Here's how the part is built. I have some questions about the finished solid (model axes, mm). Round coordinates to 2 decimals unless told otherwise and drop trailing zeros. Use a Markdown table: item, result. Add a question column.
(1) I'm going to push flat-ended pins straight in: P1, Ø5, axis at x = -11.5, y = 3.5, coming from the -Z side; P2, Ø0.9, axis at x = -13, z = -358.5, coming from the +Y side; P3, Ø1.9, axis at y = -30, z = -457.5, coming from the +X side. Where does each tip first touch, or does it pass through?
(2) If I drill on probe 1 along Y at (x, z) = (0, 13); probe 2 along Y at (x, z) = (0.75, -193); probe 3 along Y at (x, z) = (7.25, -418.5), over which ranges is the centre line in solid material (lowest first)?
(3) I want a section at A-A, the plane z = -544. Give the number of separate pieces and of enclosed holes in the cut face, then the cut area to 3 significant figures.
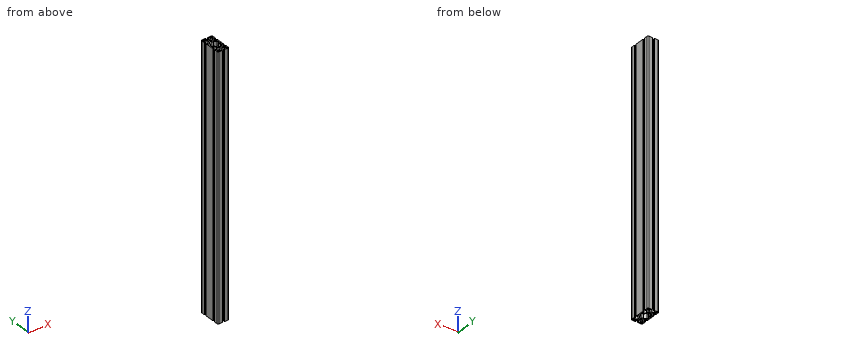
from build123d import *

# Parameters (mm, degrees)
SKETCH1_R                 = 2.45
BOSS_EXTRUDE1_DEPTH       = 700
SKETCH2_R                 = 3
CUT_EXTRUDE1_DEPTH        = 678.163200418
M6X1_0_TAPPED_HOLE1_D     = 5
M6X1_0_TAPPED_HOLE1_DEPTH = 28
M6X1_0_TAPPED_HOLE1_TIP   = 1.502151548
M6X1_0_TAPPED_HOLE2_D     = 5
M6X1_0_TAPPED_HOLE2_DEPTH = 28
M6X1_0_TAPPED_HOLE2_TIP   = 1.502151548


with BuildPart() as part:
    # Sketch1 → Boss-Extrude1 (new body)
    with BuildSketch(Plane.XY.offset(25)):
        with BuildLine():
            Line((10.271320344, -21.85), (12, -21.85))
            Line((12, -21.85), (12, -26.9))
            Line((12, -26.9), (15, -26.9))
            Line((15, -26.9), (15, -3.1))
            Line((15, -3.1), (12, -3.1))
            Line((12, -3.1), (12, -8.15))
            Line((12, -8.15), (10.271320344, -8.15))
            Line((10.271320344, -8.15), (5.25, -3.128679656))
            Line((5.25, -3.128679656), (5.25, 3.128679656))
            Line((5.25, 3.128679656), (10.271320344, 8.15))
            Line((10.271320344, 8.15), (12, 8.15))
            Line((12, 8.15), (12, 3.1))
            Line((12, 3.1), (15, 3.1))
            Line((15, 3.1), (15, 12))
            ThreePointArc((15, 12), (14.121320344, 14.121320344), (12, 15))
            Line((12, 15), (3.1, 15))
            Line((3.1, 15), (3.1, 12))
            Line((3.1, 12), (8.15, 12))
            Line((8.15, 12), (8.15, 10.271320344))
            Line((8.15, 10.271320344), (3.128679656, 5.25))
            Line((3.128679656, 5.25), (-3.128679656, 5.25))
            Line((-3.128679656, 5.25), (-8.15, 10.271320344))
            Line((-8.15, 10.271320344), (-8.15, 12))
            Line((-8.15, 12), (-3.1, 12))
            Line((-3.1, 12), (-3.1, 15))
            Line((-3.1, 15), (-12, 15))
            ThreePointArc((-12, 15), (-14.121320344, 14.121320344), (-15, 12))
            Line((-15, 12), (-15, 3.1))
            Line((-15, 3.1), (-12, 3.1))
            Line((-12, 3.1), (-12, 8.15))
            Line((-12, 8.15), (-10.271320344, 8.15))
            Line((-10.271320344, 8.15), (-5.25, 3.128679656))
            Line((-5.25, 3.128679656), (-5.25, -3.128679656))
            Line((-5.25, -3.128679656), (-10.271320344, -8.15))
            Line((-10.271320344, -8.15), (-12, -8.15))
            Line((-12, -8.15), (-12, -3.1))
            Line((-12, -3.1), (-15, -3.1))
            Line((-15, -3.1), (-15, -26.9))
            Line((-15, -26.9), (-12, -26.9))
            Line((-12, -26.9), (-12, -21.85))
            Line((-12, -21.85), (-10.271320344, -21.85))
            Line((-10.271320344, -21.85), (-5.25, -26.871320344))
            Line((-5.25, -26.871320344), (-5.25, -33.128679656))
            Line((-5.25, -33.128679656), (-10.271320344, -38.15))
            Line((-10.271320344, -38.15), (-12, -38.15))
            Line((-12, -38.15), (-12, -33.1))
            Line((-12, -33.1), (-15, -33.1))
            Line((-15, -33.1), (-15, -42))
            ThreePointArc((-15, -42), (-14.121320344, -44.121320344), (-12, -45))
            Line((-12, -45), (-3.1, -45))
            Line((-3.1, -45), (-3.1, -42))
            Line((-3.1, -42), (-8.15, -42))
            Line((-8.15, -42), (-8.15, -40.271320344))
            Line((-8.15, -40.271320344), (-3.128679656, -35.25))
            Line((-3.128679656, -35.25), (3.128679656, -35.25))
            Line((3.128679656, -35.25), (8.15, -40.271320344))
            Line((8.15, -40.271320344), (8.15, -42))
            Line((8.15, -42), (3.1, -42))
            Line((3.1, -42), (3.1, -45))
            Line((3.1, -45), (12, -45))
            ThreePointArc((12, -45), (14.121320344, -44.121320344), (15, -42))
            Line((15, -42), (15, -33.1))
            Line((15, -33.1), (12, -33.1))
            Line((12, -33.1), (12, -38.15))
            Line((12, -38.15), (10.271320344, -38.15))
            Line((10.271320344, -38.15), (5.25, -33.128679656))
            Line((5.25, -33.128679656), (5.25, -26.871320344))
            Line((5.25, -26.871320344), (10.271320344, -21.85))
        make_face()
        Circle(SKETCH1_R, mode=Mode.SUBTRACT)
        with Locations((0, -30)):
            Circle(SKETCH1_R, mode=Mode.SUBTRACT)
        with BuildLine():
            Line((-9.500000904, 12.700000174), (-9.500000904, 10.500000174))
            ThreePointArc((-9.500000904, 10.500000174), (-9.792894123, 9.792893393), (-10.500000904, 9.500000174))
            Line((-10.500000904, 9.500000174), (-12.700000904, 9.500000174))
            ThreePointArc((-12.700000904, 9.500000174), (-13.407107685, 9.792893393), (-13.700000904, 10.500000174))
            Line((-13.700000904, 10.500000174), (-13.700000904, 12.700000174))
            ThreePointArc((-13.700000904, 12.700000174), (-13.407107685, 13.407106955), (-12.700000904, 13.700000174))
            Line((-12.700000904, 13.700000174), (-10.500000904, 13.700000174))
            ThreePointArc((-10.500000904, 13.700000174), (-9.792894123, 13.407106955), (-9.500000904, 12.700000174))
        make_face(mode=Mode.SUBTRACT)
        with BuildLine():
            Line((12.700000904, 9.500000174), (10.500000904, 9.500000174))
            ThreePointArc((10.500000904, 9.500000174), (9.792894123, 9.792893393), (9.500000904, 10.500000174))
            Line((9.500000904, 10.500000174), (9.500000904, 12.700000174))
            ThreePointArc((9.500000904, 12.700000174), (9.792894123, 13.407106955), (10.500000904, 13.700000174))
            Line((10.500000904, 13.700000174), (12.700000904, 13.700000174))
            ThreePointArc((12.700000904, 13.700000174), (13.407107685, 13.407106955), (13.700000904, 12.700000174))
            Line((13.700000904, 12.700000174), (13.700000904, 10.500000174))
            ThreePointArc((13.700000904, 10.500000174), (13.407107685, 9.792893393), (12.700000904, 9.500000174))
        make_face(mode=Mode.SUBTRACT)
        with BuildLine():
            Line((-12.700000904, -39.500000174), (-10.500000904, -39.500000174))
            ThreePointArc((-10.500000904, -39.500000174), (-9.792894123, -39.792893393), (-9.500000904, -40.500000174))
            Line((-9.500000904, -40.500000174), (-9.500000904, -42.700000174))
            ThreePointArc((-9.500000904, -42.700000174), (-9.792894123, -43.407106955), (-10.500000904, -43.700000174))
            Line((-10.500000904, -43.700000174), (-12.700000904, -43.700000174))
            ThreePointArc((-12.700000904, -43.700000174), (-13.407107685, -43.407106955), (-13.700000904, -42.700000174))
            Line((-13.700000904, -42.700000174), (-13.700000904, -40.500000174))
            ThreePointArc((-13.700000904, -40.500000174), (-13.407107685, -39.792893393), (-12.700000904, -39.500000174))
        make_face(mode=Mode.SUBTRACT)
        with BuildLine():
            Line((9.500000904, -42.700000174), (9.500000904, -40.500000174))
            ThreePointArc((9.500000904, -40.500000174), (9.792894123, -39.792893393), (10.500000904, -39.500000174))
            Line((10.500000904, -39.500000174), (12.700000904, -39.500000174))
            ThreePointArc((12.700000904, -39.500000174), (13.407107685, -39.792893393), (13.700000904, -40.500000174))
            Line((13.700000904, -40.500000174), (13.700000904, -42.700000174))
            ThreePointArc((13.700000904, -42.700000174), (13.407107685, -43.407106955), (12.700000904, -43.700000174))
            Line((12.700000904, -43.700000174), (10.500000904, -43.700000174))
            ThreePointArc((10.500000904, -43.700000174), (9.792894123, -43.407106955), (9.500000904, -42.700000174))
        make_face(mode=Mode.SUBTRACT)
        Polygon((3.128679656, -24.75), (9.028679656, -18.85), (12, -18.85), (12, -11.15), (9.028679656, -11.15), (3.128679656, -5.25), (-3.128679656, -5.25), (-9.028679656, -11.15), (-12, -11.15), (-12, -18.85), (-9.028679656, -18.85), (-3.128679656, -24.75), align=None, mode=Mode.SUBTRACT)
    extrude(amount=-BOSS_EXTRUDE1_DEPTH)

    # Sketch2 → Cut-Extrude1 (cut, through all)
    with BuildSketch(Plane(origin=(15, 0, 0), x_dir=(0, 0, -1), z_dir=(1, 0, 0))):
        with Locations((30, -30)):
            Circle(SKETCH2_R)
    extrude(amount=-CUT_EXTRUDE1_DEPTH, mode=Mode.SUBTRACT)

    # M6x1.0 Tapped Hole1
    with Locations(Plane.XY.offset(25)):
        with Locations((0, 0), (0, -30)):
            Hole(M6X1_0_TAPPED_HOLE1_D / 2, depth=M6X1_0_TAPPED_HOLE1_DEPTH)
            with Locations((0, 0, -(M6X1_0_TAPPED_HOLE1_DEPTH + M6X1_0_TAPPED_HOLE1_TIP / 2))):  # 118° drill point
                Cone(0, M6X1_0_TAPPED_HOLE1_D / 2, M6X1_0_TAPPED_HOLE1_TIP, mode=Mode.SUBTRACT)

    # M6x1.0 Tapped Hole2
    with Locations(Plane(origin=(0, 0, -675), x_dir=(-1, 0, 0), z_dir=(0, 0, -1))):
        with Locations((0, 0), (0, -30)):
            Hole(M6X1_0_TAPPED_HOLE2_D / 2, depth=M6X1_0_TAPPED_HOLE2_DEPTH)
            with Locations((0, 0, -(M6X1_0_TAPPED_HOLE2_DEPTH + M6X1_0_TAPPED_HOLE2_TIP / 2))):  # 118° drill point
                Cone(0, M6X1_0_TAPPED_HOLE2_D / 2, M6X1_0_TAPPED_HOLE2_TIP, mode=Mode.SUBTRACT)


solid = part.part
Taken from the geometry:
| question | item | result |
|---|---|---|
| 1 | P1 | stops at z = -675 |
| 1 | P2 | stops at y = 14.95 |
| 1 | P3 | stops at x = 5.25 |
| 2 | probe 1 | y = -35.25 to -32.5, -27.5 to -24.75, -5.25 to -2.5, 2.5 to 5.25 |
| 2 | probe 2 | y = -35.25 to -32.33, -27.67 to -24.75, -5.25 to -2.33, 2.33 to 5.25 |
| 2 | probe 3 | y = -45 to -42, -39.37 to -35.13, -24.87 to -20.63, -9.37 to -5.13, 5.13 to 9.37, 12 to 15 |
| 3 | separate pieces | 1 |
| 3 | enclosed holes | 7 |
| 3 | area | 739 mm2 |
